from build123d import *

# Parameters (mm, degrees)
SKETCH1_R           = 2.55
BOSS_EXTRUDE1_DEPTH = 4


with BuildPart() as part:
    # Sketch1 → Boss-Extrude1 (new body)
    with BuildSketch(Plane(origin=(0, 0, 0), x_dir=(1, 0, 0), z_dir=(0, 1, 0))):
        Polygon((10, -10), (-50, -10), (-50, 10), (-10, 50), (10, 50), align=None)
        with Locations((-20, 0)):
            Circle(SKETCH1_R, mode=Mode.SUBTRACT)
        with Locations((-40, 0)):
            Circle(SKETCH1_R, mode=Mode.SUBTRACT)
        Circle(SKETCH1_R, mode=Mode.SUBTRACT)
        with Locations((0, 20)):
            Circle(SKETCH1_R, mode=Mode.SUBTRACT)
        with Locations((0, 40)):
            Circle(SKETCH1_R, mode=Mode.SUBTRACT)
    extrude(amount=BOSS_EXTRUDE1_DEPTH)


solid = part.part
Geometry: final body of the model. Coordinates: model frame, mm. Coordinates: 2 decimals unless noted, no trailing zeros. Loops run counter-clockwise (first coordinate to the right, second up) from the corner with the lowest first, then second, coordinate; pieces in that order, holes last. Notation, with made-up numbers: (30, 41.5) - (38, 41.5) arc R24 cw to (38, 59.5) - close; hole circle Ø5 at (35.25, 45). An arc over 180 degrees is marked (long way). Put each result on its own line as item: value. Start each with the question number.
Q1. Pull-direction query (Z, two-part tool) for faces 1 (the cylindrical face through (-0.33, 1.97, -42.53)), 2 (the flat face through (-30, 2, -30)), 3 (the flat face through (-13, 0, -14)); classes: released by +Z, released by -Z, zero draft, split by the parting line, or undercut.
Q2. Cut plane D-D, the plane x = -20. Return loops of the section in (y, z), and give its area (3 significant figures).
Q3. Cut plane B-B, the plane y = 2.55. Return loops of the section in (x, z).
Q4. Pin query (flat end, axial travel): pin 1 Ø6 at (x, z) = (0, -20) entering from -Y; pin 2 Ø1.5 at (y, z) = (2.5, -41.5) entering from -X. Return the tip coordinate at first contact, or that it passes through.
Q5. Cut plane C-C, the plane x = 0. Return loops of the section in (y, z), and give its area (3 significant figures).
Q6. Line query: line 1 (X direction, y = 2.15, z = 0); line 2 (Z direction, x = -2, y = 2.6). Output: solid intervals per line, ascending.
Q7. Cut plane A-A, the plane z = -40. Return loops of the section in (x, y).
Filled sheet:
1. face 1: undercut
1. face 2: released by -Z
1. face 3: zero draft
2. outline: (0, -40) - (4, -40) - (4, -2.55) - (0, -2.55) - close; (0, 2.55) - (4, 2.55) - (4, 10) - (0, 10) - close
2. area: 180 mm²
3. outline: (-50, -10) - (-10, -50) - (10, -50) - (10, 10) - (-50, 10) - close; hole circle Ø5.1 at (-40, 0); hole circle Ø5.1 at (-20, 0); hole circle Ø5.1 at (0, -40); hole circle Ø5.1 at (0, -20); hole circle Ø5.1 at (0, 0)
4. pin 1: y = 0
4. pin 2: x = -19.25
5. outline: (0, -50) - (4, -50) - (4, -42.55) - (0, -42.55) - close; (0, -37.45) - (4, -37.45) - (4, -22.55) - (0, -22.55) - close; (0, -17.45) - (4, -17.45) - (4, -2.55) - (0, -2.55) - close; (0, 2.55) - (4, 2.55) - (4, 10) - (0, 10) - close
5. area: 179 mm²
6. line 1: -50 to -42.55, -37.45 to -22.55, -17.45 to -2.55, 2.55 to 10
6. line 2: -50 to -41.58, -38.42 to -21.58, -18.42 to -1.58, 1.58 to 10
7. outline: (-20, 0) - (-2.55, 0) - (-2.55, 4) - (-20, 4) - close; (2.55, 0) - (10, 0) - (10, 4) - (2.55, 4) - close
